The figure shows three views and two pictorial views of one solid part (mm, origin at its lowest corner). Answer the questions. A direction names the side the tool comes from. Coordinates: 2 decimals unless noted, no trailing zeros. Order: outer loops, then holes, each group sorted by start corner. A loop starts at its lowest first (then second) coordinate and runs counter-clockwise, first axis right, second up. Notation, with made-up numbers: M 70.5,77.5 L 116.5,77.5 A9 cw 116.5,87.5 Z; hole C -14,-11.5 d10. An arc over 180 degrees is marked long. Use a Markdown table: item, result.
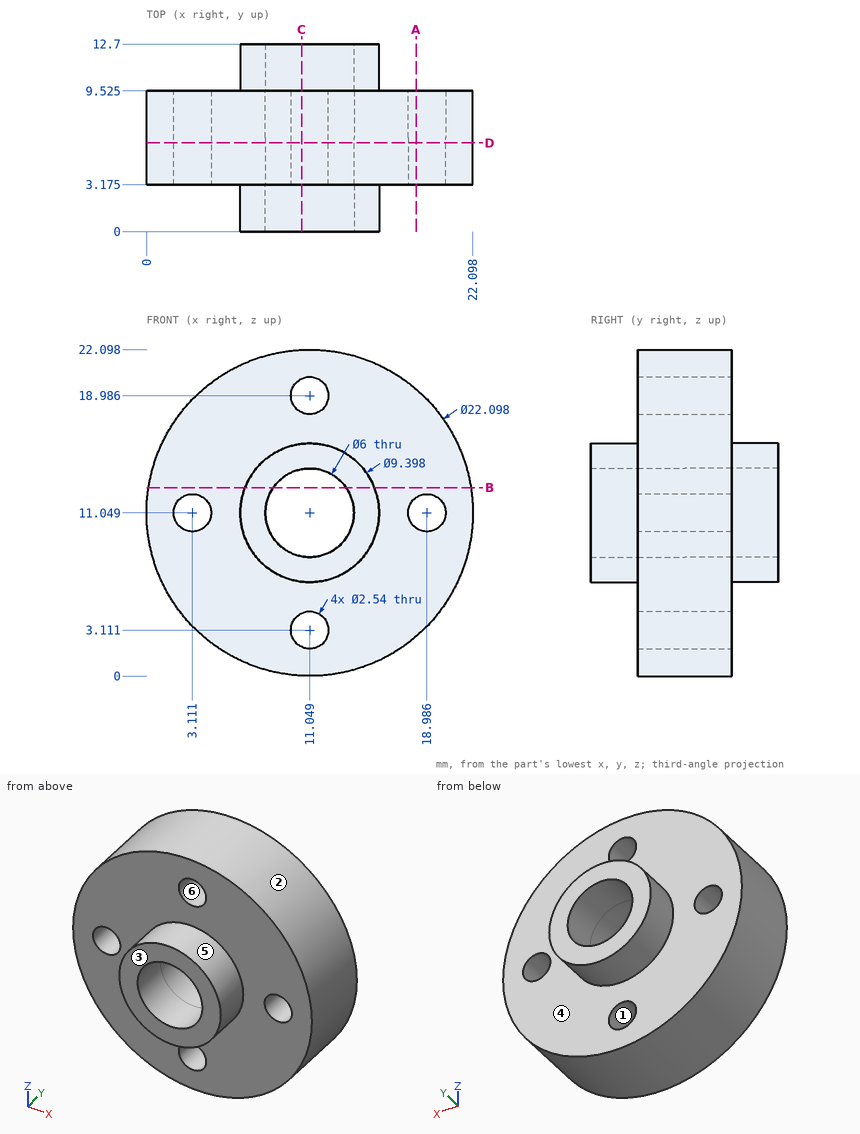
1. Section A-A on x = 18.25 is taken. Determine the outline of the cut face in (y, z) (1 decimal).
Answers below:
| item | result |
|---|---|
| outline | M 3.2,2.7 L 9.5,2.7 L 9.5,10 L 3.2,10 Z; M 3.2,12.1 L 9.5,12.1 L 9.5,19.4 L 3.2,19.4 Z |
2. For a pull along X with two mould halves and no side action, classify the marked faces 1, 2 and 3 as +X half, -X half, draft (parallel to the pull), parting line (faces both ways), or undercut.
Answers below:
| item | result |
|---|---|
| face 1 | undercut |
| face 2 | parting line |
| face 3 | draft |
3. Section D-D on y = 6 is taken. Determine the outline of the cut face in (x, z), then the cut area to 3 significant figures.
Answers below:
| item | result |
|---|---|
| outline | C 11.05,11.05 d22.1; hole C 3.11,11.05 d2.54; hole C 11.05,11.05 d6; hole C 11.05,3.11 d2.54; hole C 11.05,18.99 d2.54; hole C 18.99,11.05 d2.54 |
| area | 335 mm² |
4. Section B-B on z = 12.75 is taken. Determine the outline of the cut face in (x, y) (1 decimal).
Answers below:
| item | result |
|---|---|
| outline | M 0.1,3.2 L 6.7,3.2 L 6.7,0 L 8.6,0 L 8.6,12.7 L 6.7,12.7 L 6.7,9.5 L 0.1,9.5 Z; M 13.5,0 L 15.4,0 L 15.4,3.2 L 22,3.2 L 22,9.5 L 15.4,9.5 L 15.4,12.7 L 13.5,12.7 Z |
5. Find the intervals of material crossed by probe 1 along Z at (x, y) = (11.25, 3) (1 decimal); probe 2 along Y at (x, z) = (13.75, 17) (1 decimal); probe 3 along X at (y, z) = (7.25, 8.75) (1 decimal), in increasing order.
Answers below:
| item | result |
|---|---|
| probe 1 | 6.4 to 8.1, 14 to 15.7 |
| probe 2 | 3.2 to 9.5 |
| probe 3 | 0.2 to 9.1, 13 to 21.9 |
6. Flat-ended cylindrical pins translate along their axes: P1, Ø1.5, axis at x = 15, z = 4, coming from the +Y side (1 decimal); P2, Ø3, axis at y = 6.5, z = 20, coming from the +X side; P3, Ø3.5, axis at x = 11.05, z = 3.11, coming from the -Y side (1 decimal). Find the tip coordinate at first contact, or state that the pin passes through.
Answers below:
| item | result |
|---|---|
| P1 | y = 9.5 |
| P2 | x = 19.21 |
| P3 | y = 3.2 |
7. Section C-C on x = 10.5 is taken. Determine the outline of the cut face in (y, z) (1 decimal).
Answers below:
| item | result |
|---|---|
| outline | M 0,6.4 L 3.2,6.4 L 3.2,4.3 L 9.5,4.3 L 9.5,6.4 L 12.7,6.4 L 12.7,8.1 L 0,8.1 Z; M 0,14 L 12.7,14 L 12.7,15.7 L 9.5,15.7 L 9.5,17.8 L 3.2,17.8 L 3.2,15.7 L 0,15.7 Z; M 3.2,0 L 9.5,0 L 9.5,2 L 3.2,2 Z; M 3.2,20.1 L 9.5,20.1 L 9.5,22.1 L 3.2,22.1 Z |
8. For the marked faces 4, 5 and 6, determine the directions among +Z, -Z, +X, -X, +Y, -Y from which every point of the face is accessible in a straight line to the end or side of a thin tool.
Answers below:
| item | result |
|---|---|
| face 4 | +Y |
| face 5 | -Y |
| face 6 | +Y, -Y |
